```python
from build123d import *

# Parameters (mm, degrees)
F1_DEPTH = 2.5
F2_R     = 2


with BuildPart() as f1:
    # F0 (on Top) → F1 (new body)
    with BuildSketch(Plane.XY):
        with BuildLine():
            Line((-8.0375, 13.921358), (-9.5, 16.454483))
            ThreePointArc((-9.5, 16.454483), (-18.831831, 2.522325), (-13.495278, -13.374508))
            ThreePointArc((-13.495278, -13.374508), (-9.5, -16.454483), (-4.835024, -18.374508))
            ThreePointArc((-4.835024, -18.374508), (11.600313, -15.047682), (19, 0))
            Line((19, 0), (16.075, 0))
            ThreePointArc((16.075, 0), (-8.0375, -13.921358), (-8.0375, 13.921358))
        make_face()
        with BuildLine():
            ThreePointArc((-4.835024, -18.374508), (-9.5, -16.454483), (-13.495278, -13.374508))
            Line((-13.495278, -13.374508), (-13.830127, -13.954483))
            Line((-13.830127, -13.954483), (-14.830127, -15.686533))
            Line((-14.830127, -15.686533), (-16.562178, -14.686533))
            Line((-16.562178, -14.686533), (-17.062178, -15.552559))
            ThreePointArc((-17.062178, -15.552559), (-11.543396, -19.993749), (-4.937822, -22.552559))
            Line((-4.937822, -22.552559), (-4.437822, -21.686533))
            Line((-4.437822, -21.686533), (-6.169873, -20.686533))
            Line((-6.169873, -20.686533), (-5.169873, -18.954483))
            Line((-5.169873, -18.954483), (-4.835024, -18.374508))
        make_face()
    extrude(amount=F1_DEPTH)

    # F2
    f2_edges = [f1.edges().sort_by_distance(p)[0] for p in [
        (19, 0, 1.25),
        (-9.5, 16.454483, 1.25),
    ]]
    fillet(f2_edges, radius=F2_R)


solid = f1.part
```
Can you work these out from the model? Positions are in its coordinate system, mm. A direction names the side the tool comes from. Coordinates: 2 decimals unless noted, no trailing zeros. Write each loop counter-clockwise with the first axis right and the second up, starting at its lowest first coordinate (ties: lowest second). Pieces come first, ordered by that corner, then holes. Notation, with made-up numbers: M 8.5,-5 L 22.5,-5 A33 cw 22.5,24 Z; hole C -37.5,7.5 d7. An arc over 180 degrees is marked long. Answer as CSV lines item,"result".
Item 1: Please list where these lines run through material, in increasing order: line 1 along X through (y, z) = (-11, 2.2); line 2 along Y through (x, z) = (0, 0.5) (3 decimals); line 3 along X through (y, z) = (-6.5, 1.8).
Geometry results:
line 1,"x = -15.49 to -11.72, 11.72 to 15.49"
line 2,"y = -19 to -16.075"
line 3,"x = -17.85 to -14.7, 14.7 to 17.85"
Item 2: We'd pull the mould along X, two halves only. Please class faces 3 (the flat face through (-7, -15, 2.5)), 4 (the flat face through (-15.684, -15.194, 1.232)), 5 (the flat face through (-16.8, -15.1, 1.2)): +X half, -X half, draft (parallel to the pull), parting line (faces both ways), or undercut.
Geometry results:
face 3,"draft"
face 4,"undercut"
face 5,"-X half"
Item 3: I'm going to push flat-ended pins straight in: P1, Ø0.9, axis at x = 16.5, z = 1, coming from the +Y side; P2, Ø1, axis at y = 1, z = 1, coming from the +X side. Where does each tip first touch, or does it pass through?
Geometry results:
P1,"stops at y = 0"
P2,"stops at x = -16"
Item 4: On a 3-axis mill with a long thin cutter (end or side, diameter ignored), from which of +Z, -Z, +X, -X, +Y, -Y can I reach the whole of each face in a straight line? I mean faces 1 (the flat face through (-5.292, -21.194, 1.232)), 2 (the cylindrical face through (-18.93, 1.63, 1.23)). Say none if no direction works.
Geometry results:
face 1,"+Z, -Z, +X"
face 2,"+Z, -Z, -X"
Item 5: Imagine slicing it at B-B on y = -5.5. List the corners of the cut face in (x, z) for me, plus the area to 3 significant figures.
Geometry results:
outline,"M -18.19,0 L -15.1,0 L -15.1,2.5 L -18.19,2.5 Z; M 15.1,0 L 18.19,0 L 18.19,2.5 L 15.1,2.5 Z"
area,"15.4 mm2"
Item 6: Imagine slicing it at D-D on x = 3. List the corners of the cut face in (y, z) for me.
Geometry results:
outline,"M -18.76,0 L -15.79,0 L -15.79,2.5 L -18.76,2.5 Z"
Item 7: Imagine slicing it at C-C on x = -9. List the corners of the cut face in (y, z) for me.
Geometry results:
outline,"M -21.26,0 L -13.32,0 L -13.32,2.5 L -21.26,2.5 Z; M 13.32,0 L 15.24,0 L 15.24,2.5 L 13.32,2.5 Z"
